from build123d import *

# Parameters (mm, degrees)
CROQUIS1_W              = 65
CROQUIS1_H              = 28
SALIENTE_EXTRUIR1_DEPTH = 8
CROQUIS2_W              = 8
CROQUIS2_H              = 28
SALIENTE_EXTRUIR2_DEPTH = 28
CROQUIS3_R              = 14
SALIENTE_EXTRUIR3_DEPTH = 8
CROQUIS4_R              = 14
SALIENTE_EXTRUIR4_DEPTH = 8
CROQUIS5_R              = 11.115
CORTAR_EXTRUIR1_DEPTH   = 5
CROQUIS6_R              = 5.155
CORTAR_EXTRUIR2_DEPTH   = 8
CORTAR_EXTRUIR3_START   = -8
CROQUIS7_R              = 6.5
CORTAR_EXTRUIR3_DEPTH   = 5
CROQUIS8_R              = 1.5
CORTAR_EXTRUIR4_DEPTH   = 8


with BuildPart() as part:
    # Croquis1 → Saliente-Extruir1 (new body)
    with BuildSketch(Plane.XY):
        with Locations((32.5, 14)):
            Rectangle(CROQUIS1_W, CROQUIS1_H)
    extrude(amount=SALIENTE_EXTRUIR1_DEPTH)

    # Croquis2 → Saliente-Extruir2 (add)
    with BuildSketch(Plane.XY.offset(8)):
        with Locations((4, 14)):
            Rectangle(CROQUIS2_W, CROQUIS2_H)
        with Locations((61, 14)):
            Rectangle(CROQUIS2_W, CROQUIS2_H)
    extrude(amount=SALIENTE_EXTRUIR2_DEPTH)

    # Croquis3 → Saliente-Extruir3 (add)
    with BuildSketch(Plane.ZY):
        with Locations((36, 14)):
            Circle(CROQUIS3_R)
    extrude(amount=-SALIENTE_EXTRUIR3_DEPTH)

    # Croquis4 → Saliente-Extruir4 (add)
    with BuildSketch(Plane(origin=(65, 0, 0), x_dir=(0, 0, -1), z_dir=(1, 0, 0))):
        with Locations((-36, 14)):
            Circle(CROQUIS4_R)
    extrude(amount=-SALIENTE_EXTRUIR4_DEPTH)

    # Croquis5 → Cortar-Extruir1 (cut)
    with BuildSketch(Plane.ZY):
        with Locations((36, 14)):
            Circle(CROQUIS5_R)
    extrude(amount=-CORTAR_EXTRUIR1_DEPTH, mode=Mode.SUBTRACT)

    # Croquis6 → Cortar-Extruir2 (cut)
    with BuildSketch(Plane.ZY):
        with Locations((36, 14)):
            Circle(CROQUIS6_R)
    extrude(amount=-CORTAR_EXTRUIR2_DEPTH, mode=Mode.SUBTRACT)

    # Croquis7 → Cortar-Extruir3 (cut)
    with BuildSketch(Plane(origin=(65, 0, 0), x_dir=(0, 0, -1), z_dir=(1, 0, 0)).offset(CORTAR_EXTRUIR3_START)):
        with Locations((-36, 14)):
            Circle(CROQUIS7_R)
    extrude(amount=CORTAR_EXTRUIR3_DEPTH, mode=Mode.SUBTRACT)

    # Croquis8 → Cortar-Extruir4 (cut)
    with BuildSketch(Plane.XY.offset(8)):
        with Locations((39.5, 21)):
            Circle(CROQUIS8_R)
        with Locations((25.5, 21)):
            Circle(CROQUIS8_R)
        with Locations((25.5, 7)):
            Circle(CROQUIS8_R)
        with Locations((39.5, 7)):
            Circle(CROQUIS8_R)
    extrude(amount=-CORTAR_EXTRUIR4_DEPTH, mode=Mode.SUBTRACT)


solid = part.part
Input: part model. Units: mm. Frame: model coordinates. A direction names the side the tool comes from. Give positions to 0.01 mm unless a question says otherwise; leave off trailing zeros. Order: outer loops, then holes, each group sorted by start corner. A loop starts at its lowest first (then second) coordinate and runs counter-clockwise, first axis right, second up. Notation, with made-up numbers: (24, -32) - (55, -32) arc R7 cw to (55, -23) - close; hole circle Ø3 at (37.5, -10). An arc over 180 degrees is marked (long way). Answer as a JSON object with one key per item and string values. Group by question number.
Q1. Cut plane A-A, the plane z = 21. Output: boundary loops of the cut face in (x, y), then the cut area to 3 significant figures.
Q2. Cut plane D-D, the plane x = 60.5. Output: boundary loops of the cut face in (y, z), then the cut area to 3 significant figures.
Q3. Line query: probe 1 along Y at (x, z) = (25.5, 4); probe 2 along X at (y, z) = (5.75, 17.5); probe 3 along Y at (x, z) = (6, 36) (3 decimals). Output: solid intervals per line, ascending.
Q4. Cut plane C-C, the plane y = 16.5. Output: boundary loops of the cut face in (x, z), then the cut area to 3 significant figures.
Q5. Set-up query: faces 1 (the face through (8, 14, 29)), 2 (the face through (2.465, 9.743, 46.267)), 3 (the face through (62, 14, 36)). Return all of +Z, -Z, +X, -X, +Y, -Y with unobstructed straight access to the full face (end or side cutting, diameter ignored); none if empty.
Q6. First-contact query: pin 1 Ø1.8 at (x, y) = (25.5, 21) entering from +Z; pin 2 Ø14 at (x, y) = (40.5, 9.5) entering from +Z; pin 3 Ø3 at (y, z) = (21, 11.5) entering from -X; pin 4 Ø5 at (y, z) = (17, 32) entering from -X. Flat tips, straight axial feed; report the tip coordinate or a pass-through.
Q7. Mould query, pull axis Y, two halves, no side actions, for faces 4 (the face through (24, 7, 4)), 5 (the face through (32, 0, 6)), 6 (the face through (32, 14, 8)), 7 (the face through (6.479, 15.548, 40.917)). Classes: pulls with the +Y half, pulls with the -Y half, needs draft (parallel to the pull), parting line crosses it, or undercut.
Q8. Cut plane B-B, the plane x = 25.5. Output: boundary loops of the cut face in (y, z), then the cut area to 3 significant figures.
Results:
{
 "1": {"outline": "(0, 0) - (8, 0) - (8, 28) - (0, 28) - close; (57, 0) - (65, 0) - (65, 28) - (57, 28) - close", "area": "448 mm^2"},
 "2": {"outline": "(0, 0) - (28, 0) - (28, 36) arc R14 ccw to (0, 36) - close; hole circle Ø13 at (14, 36)", "area": "1,180 mm^2"},
 "3": {"probe 1": "0 to 5.5, 8.5 to 19.5, 22.5 to 28", "probe 2": "0 to 8, 57 to 65", "probe 3": "0 to 8.845, 19.155 to 28"},
 "4": {"outline": "(0, 0) - (65, 0) - (65, 49.77) - (57, 49.77) - (57, 42) - (62, 42) - (62, 30) - (57, 30) - (57, 8) - (8, 8) - (8, 31.49) - (5, 31.49) - (5, 25.17) - (0, 25.17) - close; (0, 46.83) - (5, 46.83) - (5, 40.51) - (8, 40.51) - (8, 49.77) - (0, 49.77) - close", "area": "993 mm^2"},
 "5": {"face 1": "+Z, +Y, -Y", "face 2": "-X", "face 3": "none"},
 "6": {"pin 1": "through", "pin 2": "z = 8", "pin 3": "x = 0", "pin 4": "x = 5"},
 "7": {"face 4": "undercut", "face 5": "pulls with the -Y half", "face 6": "needs draft", "face 7": "undercut"},
 "8": {"outline": "(0, 0) - (5.5, 0) - (5.5, 8) - (0, 8) - close; (8.5, 0) - (19.5, 0) - (19.5, 8) - (8.5, 8) - close; (22.5, 0) - (28, 0) - (28, 8) - (22.5, 8) - close", "area": "176 mm^2"}
}
